Could you check a few things on this model? Use its own coordinates, in mm. Face numbers are marked on the shaded views. Give positions to 0.01 mm unless a question says otherwise; leave off trailing zeros. Order: outer loops, then holes, each group sorted by start corner. A loop starts at its lowest first (then second) coordinate and runs counter-clockwise, first axis right, second up. Notation, with made-up numbers: (49, 84) -> (57, 84) arc R18 cw to (57, 106) -> close; hole circle Ø4 at (25.5, 13). An arc over 180 degrees is marked (long way). Use one line per item in the form item = value. Start each with the question number.
Autodesk Inventor part; units mm, degrees
ref_plane "YZ Plane" through (0, 0, 0) normal (1, 0, 0) x (0, 1, 0)
ref_plane "XZ Plane" through (0, 0, 0) normal (0, 1, 0) x (-1, 0, 0)
ref_plane "XY Plane" through (0, 0, 0) normal (0, 0, 1) x (1, 0, 0)
sketch "Sketch1" plane through (0, 0, 0) normal (0, 1, 0) x (-1, 0, 0)
  circle A0 centre (0, 0) radius 33.995
  circle A1 centre (0, 0) radius 5.005
  dimension "d0" = 67.99
  dimension "d1" = 10.01
extrude "Extrusion1" add sketch "Sketch1" along normal blind 70
sketch "Sketch2" plane through (0, 0, 0) normal (0, -1, 0) x (1, 0, 0)
  circle A0 centre (0, 0) radius 5.005
  circle A1 centre (0, 0) radius 10.005
  dimension "d4" = 20.01
extrude "Extrusion2" cut sketch "Sketch2" against normal blind 50
sketch "Sketch3" plane through (0, 70, 0) normal (0, 1, 0) x (1, 0, 0)
  circle A0 centre (0, 0) radius 7.5
  dimension "d7" = 15
extrude "Extrusion3" cut sketch "Sketch3" against normal blind 1
fillet "Fillet1" radius 0.5 1 edges at (-7.5, 70, 0)
properties part number "top" material "Steel, Mild"
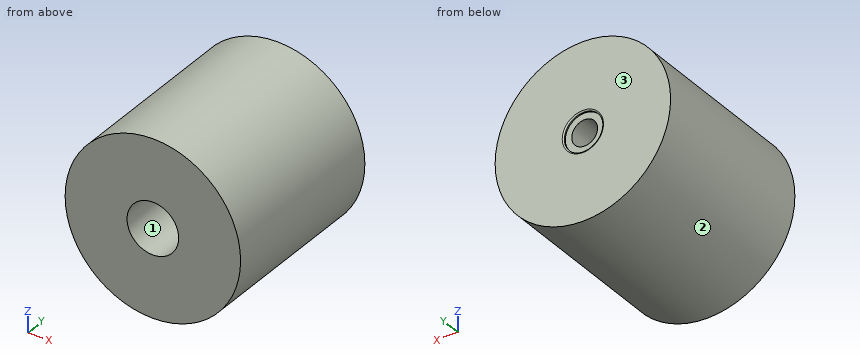
(1) I'm going to push flat-ended pins straight in: pin 1 Ø5 at (x, y) = (-17.5, 52.5) entering from -Z; pin 2 Ø3 at (x, y) = (18.5, 12.5) entering from -Z; pin 3 Ø8 at (x, z) = (0, 0) entering from -Y; pin 4 Ø5 at (y, z) = (26.5, 9.5) entering from -X. Where does each tip first touch, or does it pass through?
(2) Imagine slicing it at C-C (y = 32). Write out the boundary of the cut face in (x, z) (3 decimals).
(3) Imagine slicing it at D-D (x = 11.5). Write out the boundary of the cut face in (y, z).
(4) We'd pull the mould along X, two halves only. Please class the marked faces 1, 2 and 3: pulls with the +X half, pulls with the -X half, needs draft (parallel to the pull), parting line crosses it, or undercut.
(5) Please list where these lines run through material, in increasing order: probe 1 along Z at (x, y) = (0, 69.35) (3 decimals); probe 2 along Z at (x, y) = (0, 25) (3 decimals); probe 3 along X at (y, z) = (49, -2).
(6) Imagine slicing it at B-B (z = 0). Write out the boundary of the cut face in (x, y) (3 decimals), plus the area to 3 significant figures.
(7) Imagine slicing it at A-A (x = 0). Write out the boundary of the cut face in (y, z) (3 decimals).
Calculated:
q1.pin_1 = -30.51
q1.pin_2 = -29.44
q1.pin_3 = through
q1.pin_4 = -33.27
q2.outline = circle Ø67.99 at (0, 0); hole circle Ø20.01 at (0, 0)
q3.outline = (0, -31.99) -> (70, -31.99) -> (70, 31.99) -> (0, 31.99) -> close
q4.face_1 = undercut
q4.face_2 = parting line crosses it
q4.face_3 = needs draft
q5.probe_1 = -33.995 to -7.5, 7.5 to 33.995
q5.probe_2 = -33.995 to -10.005, 10.005 to 33.995
q5.probe_3 = -33.94 to -9.8, 9.8 to 33.94
q6.outline = (-33.995, 0) -> (-10.005, 0) -> (-10.005, 50) -> (-5.005, 50) -> (-5.005, 69) -> (-7.5, 69) -> (-7.5, 69.5) arc R0.5 ccw to (-8, 70) -> (-33.995, 70) -> close; (5.005, 50) -> (10.005, 50) -> (10.005, 0) -> (33.995, 0) -> (33.995, 70) -> (8, 70) arc R0.5 ccw to (7.5, 69.5) -> (7.5, 69) -> (5.005, 69) -> close
q6.area = 3,550 mm2
q7.outline = (0, -33.995) -> (70, -33.995) -> (70, -8) arc R0.5 ccw to (69.5, -7.5) -> (69, -7.5) -> (69, -5.005) -> (50, -5.005) -> (50, -10.005) -> (0, -10.005) -> close; (0, 10.005) -> (50, 10.005) -> (50, 5.005) -> (69, 5.005) -> (69, 7.5) -> (69.5, 7.5) arc R0.5 ccw to (70, 8) -> (70, 33.995) -> (0, 33.995) -> close
